Autodesk Inventor part; units mm, degrees
ref_plane "Work Plane1" through (0, 16, 0) normal (0, 1, 0) x (1, 0, 0)
ref_plane "YZ Plane" through (0, 0, 0) normal (1, 0, 0) x (0, 1, 0)
ref_plane "XZ Plane" through (0, 0, 0) normal (0, 1, 0) x (-1, 0, 0)
sketch "Sketch1" plane through (0, 0, 0) normal (0, 1, 0) x (-1, 0, 0)
  circle A0 centre (0, 0) radius 4
  dimension "d0" = 8
extrude "Extrusion1" add sketch "Sketch1" along normal blind 36
sketch "Sketch3" plane through (0, 0, 0) normal (0, -1, 0) x (1, 0, 0)
  line L0 (-1.1832, 0.85) -> (1.1832, 0.85)
  arc A0 (-1.1832, 0.85) -> (1.1832, 0.85) centre (0, 0.2) ccw
  point P0 (0, 0)
  point P1 (0, 0)
  point P2 (0, 0.85)
  dimension "d16" = 1.35
  dimension "d17" = 0.2
  dimension "d39" = 2
extrude "Extrusion3" add sketch "Sketch3" along normal blind 15.25
sketch "Sketch5" plane through (0, 0, 0) normal (0, -1, 0) x (1, 0, 0)
  circle A0 centre (0, 0) radius 5.5
  dimension "d29" = 11
extrude "Extrusion5" add sketch "Sketch5" against normal blind 2
chamfer "Chamfer3" distance 0.5 angle 45 2 edges at (-5.5, 0, 0) (-5.5, 2, 0)
sketch "Sketch6" plane through (0, 0, 0) normal (0, -1, 0) x (1, 0, 0)
  circle A0 centre (0, 0) radius 5
  line L0 (-7.7, 0) -> (7.7, 0)
  line L1 (0, -7.7) -> (0, 7.7)
  circle A1 centre (0, 0) radius 4
  dimension "d35" = 8
extrude "Extrusion6" add sketch "Sketch6" along normal blind 4 contours A1 L1 L0 | L0 L1 A1 | L1 L0 A1 | A1 L0 L1
ref_plane "Work Plane1" through (0, 16, 0) normal (0, 1, 0) x (1, 0, 0)
mirror "Mirror1" about plane through (0, 16, 0) normal (0, 1, 0) of "Extrusion3"
properties part number "axle-skibidi"
Could you check a few things on this model? Use its own coordinates, in mm. A direction names the side the tool comes from. Round coordinates to 2 decimals unless told otherwise and drop trailing zeros. Loops run counter-clockwise (first coordinate to the right, second up) from the corner with the lowest first, then second, coordinate; pieces in that order, holes last. Notation, with made-up numbers: (-39.5, 82.5) -> (-13.5, 82.5) arc R27 cw to (-13.5, 115.5) -> close; hole circle Ø5 at (37, -33). An arc over 180 degrees is marked (long way). Put each result on its own line as item: value.
Q1. Please list where these lines run through material, in increasing order: line 1 (Y direction, x = 4.75, z = 0); line 2 (Y direction, x = -2, z = 1.5); line 3 (X direction, y = 15.5, z = -3.5). Write a range as from..to.
Checks:
line 1: 0..2
line 2: -4..36
line 3: -1.94..1.94
Q2. For pin 1 Ø4 at (y, z) = (14, 3) entering from +X; pin 2 Ø3 at (y, z) = (22.5, 4) entering from -X; pin 3 Ø3 at (x, z) = (-0.5, -1.5) entering from +Y; pin 4 Ø6 at (x, z) = (-4, 3) entering from -Y, each with a flat end and sliding along its axis, tell me the tip position at first contact or that it passes through.
Checks:
pin 1: x = 3.87
pin 2: x = -3.12
pin 3: y = 47.25
pin 4: y = -4
Q3. I want a section at C-C on z = 0. Write out the boundary of the cut face in (x, y), and give its area (3 significant figures).
Checks:
outline: (-5.5, 0.5) -> (-5, 0) -> (-4, 0) -> (-4, -4) -> (-1.34, -4) -> (-1.34, -15.25) -> (1.34, -15.25) -> (1.34, -4) -> (4, -4) -> (4, 0) -> (5, 0) -> (5.5, 0.5) -> (5.5, 1.5) -> (5, 2) -> (4, 2) -> (4, 36) -> (1.34, 36) -> (1.34, 47.25) -> (-1.34, 47.25) -> (-1.34, 36) -> (-4, 36) -> (-4, 2) -> (-5, 2) -> (-5.5, 1.5) -> close
area: 386 mm2
Q4. I want a section at A-A on x = 0. Write out the boundary of the cut face in (y, z), and give its area (4 significant figures).
Checks:
outline: (-15.25, -1.15) -> (-4, -1.15) -> (-4, -4) -> (0, -4) -> (0, -5) -> (0.5, -5.5) -> (1.5, -5.5) -> (2, -5) -> (2, -4) -> (36, -4) -> (36, -1.15) -> (47.25, -1.15) -> (47.25, 0.85) -> (36, 0.85) -> (36, 4) -> (2, 4) -> (2, 5) -> (1.5, 5.5) -> (0.5, 5.5) -> (0, 5) -> (0, 4) -> (-4, 4) -> (-4, 0.85) -> (-15.25, 0.85) -> close
area: 370.5 mm2
Q5. I want a section at B-B on y = -9. Write out the boundary of the cut face in (x, z).
Checks:
outline: (-1.18, 0.85) arc R1.35 ccw (long way) to (1.18, 0.85) -> close
Q6. Which directions (+Z, -Z, +X, -X, +Y, -Y) give clear straight access to the entire face, cutting with the end or side of a thin tool? Please do faces 1 (the flat face through (0, 42, 0.85)), 2 (the cylindrical face through (-0.04, 41.55, -1.15)), 3 (the cylindrical face through (0.04, -9.55, -1.15)).
Checks:
face 1: +Z, +X, -X, +Y
face 2: +Y
face 3: -Y
Q7. I want a section at D-D on y = 26.5. Write out the boundary of the cut face in (x, z).
Checks:
outline: circle Ø8 at (0, 0)
